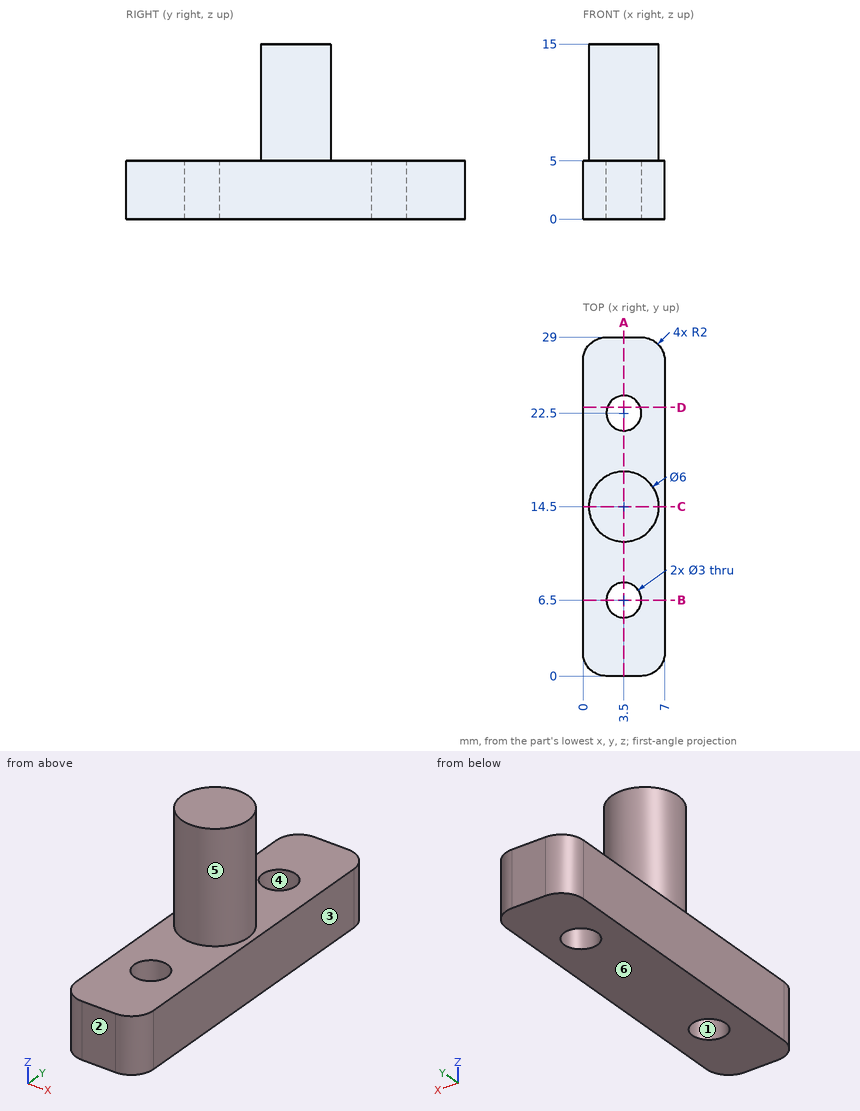
Geometry: see drawing. Coordinates: mm, zero at the bounding-box minimum. A direction names the side the tool comes from. Give positions to 0.01 mm unless a question says otherwise; leave off trailing zeros. Loops run counter-clockwise (first coordinate to the right, second up) from the corner with the lowest first, then second, coordinate; pieces in that order, holes last. Notation, with made-up numbers: (39.5, 72) - (80.5, 72) arc R24 ccw to (80.5, 110) - close; hole circle Ø7 at (20.5, -8). An arc over 180 degrees is marked (long way). Use CSV: the item, a comma, the result in double quotes. Start each with the question number.
1. Reachability of the marked faces 5 and 6 from +Z, -Z, +X, -X, +Y, -Y: full face, straight path, thin tool, end or side. Return the list, or none.
2. Section A-A (x = 3.5). Output: boundary loops of the cut face in (y, z).
3. Ray query, L1, parallel to Y at x = 3.5, z = 1.2; L2, parallel to Z at x = 5, y = 25; L3, parallel to Y at x = 6.25, z = 1. Return the intervals inside material, ascending.
4. Draft query along X for the marked faces 1, 2, 3 and 4. Return one class per face: +X half, -X half, draft (parallel to the pull), parting line (faces both ways), or undercut.
5. Section C-C (y = 14.5). Output: boundary loops of the cut face in (x, z), then the cut area to 3 significant figures.
6. Section B-B (y = 6.5). Output: boundary loops of the cut face in (x, z), then the cut area to 3 significant figures.
7. Pin query (flat end, axial travel): pin 1 (4 mm diameter, centred on x = 1.5, z = 1.5, fed in from -Y); pin 2 (2.5 mm diameter, centred on x = 3.5, y = 22.5, fed in from -Z); pin 3 (3 mm diameter, centred on y = 13.5, z = 9, fed in from +X); pin 4 (1 mm diameter, centred on x = 6, z = 4.5, fed in from +Y). Return the tip coordinate at first contact, or that it passes through.
8. Section D-D (y = 23). Output: boundary loops of the cut face in (x, z), then the cut area to 3 significant figures.
Response:
1,face 5,"+Z"
1,face 6,"-Z, +X, -X, +Y, -Y"
2,outline,"(0, 0) - (5, 0) - (5, 5) - (0, 5) - close; (8, 0) - (21, 0) - (21, 5) - (17.5, 5) - (17.5, 15) - (11.5, 15) - (11.5, 5) - (8, 5) - close; (24, 0) - (29, 0) - (29, 5) - (24, 5) - close"
3,L1,"0 to 5, 8 to 21, 24 to 29"
3,L2,"0 to 5"
3,L3,"0.44 to 28.56"
4,face 1,"undercut"
4,face 2,"draft"
4,face 3,"+X half"
4,face 4,"undercut"
5,outline,"(0, 0) - (7, 0) - (7, 5) - (6.5, 5) - (6.5, 15) - (0.5, 15) - (0.5, 5) - (0, 5) - close"
5,area,"95.0 mm²"
6,outline,"(0, 0) - (2, 0) - (2, 5) - (0, 5) - close; (5, 0) - (7, 0) - (7, 5) - (5, 5) - close"
6,area,"20.0 mm²"
7,pin 1,"y = 0"
7,pin 2,"through"
7,pin 3,"x = 6.5"
7,pin 4,"y = 28.94"
8,outline,"(0, 0) - (2.09, 0) - (2.09, 5) - (0, 5) - close; (4.91, 0) - (7, 0) - (7, 5) - (4.91, 5) - close"
8,area,"20.9 mm²"
